The listing builds one solid part. Answer for the finished solid, in the listing's coordinates (mm). A direction names the side the tool comes from. Give positions to 0.01 mm unless a question says otherwise; leave off trailing zeros. Write each loop counter-clockwise with the first axis right and the second up, starting at its lowest first coordinate (ties: lowest second). Pieces come first, ordered by that corner, then holes. Notation, with made-up numbers: M 82.5,36.5 L 114.5,36.5 A14 cw 114.5,51.5 Z; hole C 27,81 d2. An arc over 180 degrees is marked long. Answer as a JSON object with one key per item and string values.
```python
from build123d import *

# Parameters (mm, degrees)
F1_DEPTH = 11
F2_R     = 28.523991
F3_R     = 5
F5_R     = 0.75
F6_DEPTH = 11.001
F7_R     = 4
F8_DEPTH = 11.001


with BuildPart() as f1:
    # F0 (on Top) → F1 (new body)
    with BuildSketch(Plane.XY):
        with BuildLine():
            ThreePointArc((-59.119348, -199.42142), (-183.034682, -98.804378), (-199.158229, 60))
            Line((-199.158229, 60), (-222.036033, 60))
            ThreePointArc((-222.036033, 60), (0, -230), (222.036033, 60))
            Line((222.036033, 60), (199.158229, 60))
            ThreePointArc((199.158229, 60), (183.034682, -98.804378), (59.119348, -199.42142))
            Line((59.119348, -199.42142), (25, -188))
            Line((25, -188), (0, -188))
            Line((0, -188), (-25, -188))
            Line((-25, -188), (-59.119348, -199.42142))
        make_face()
    extrude(amount=F1_DEPTH)

    # F2
    f2_edges = [f1.edges().sort_by_distance(p)[0] for p in [
        (25, -188, 5.5),
        (-25, -188, 5.5),
    ]]
    fillet(f2_edges, radius=F2_R)

    # F3
    f3_edges = [f1.edges().sort_by_distance(p)[0] for p in [
        (59.119348, -199.42142, 5.5),
        (-59.119348, -199.42142, 5.5),
    ]]
    fillet(f3_edges, radius=F3_R)

    # F5 (on face) → F6 (cut, through all)
    with BuildSketch(Plane.XY.offset(11)):
        with Locations((0, -219)):
            Circle(F5_R)
        with Locations((48.732085, -213.509213)):
            Circle(F5_R)
        with Locations((95.020539, -197.312182)):
            Circle(F5_R)
        with Locations((136.544267, -171.221095)):
            Circle(F5_R)
        with Locations((171.221095, -136.544267)):
            Circle(F5_R)
        with Locations((197.312182, -95.020539)):
            Circle(F5_R)
        with Locations((213.509213, -48.732085)):
            Circle(F5_R)
        with Locations((219, 0)):
            Circle(F5_R)
        with Locations((213.509213, 48.732085)):
            Circle(F5_R)
        with Locations((197.312182, 95.020539)):
            Circle(F5_R)
        with Locations((171.221095, 136.544267)):
            Circle(F5_R)
        with Locations((136.544267, 171.221095)):
            Circle(F5_R)
        with Locations((95.020539, 197.312182)):
            Circle(F5_R)
        with Locations((48.732085, 213.509213)):
            Circle(F5_R)
        with Locations((0, 219)):
            Circle(F5_R)
        with Locations((-48.732085, 213.509213)):
            Circle(F5_R)
        with Locations((-95.020539, 197.312182)):
            Circle(F5_R)
        with Locations((-136.544267, 171.221095)):
            Circle(F5_R)
        with Locations((-171.221095, 136.544267)):
            Circle(F5_R)
        with Locations((-197.312182, 95.020539)):
            Circle(F5_R)
        with Locations((-213.509213, 48.732085)):
            Circle(F5_R)
        with Locations((-219, 0)):
            Circle(F5_R)
        with Locations((-213.509213, -48.732085)):
            Circle(F5_R)
        with Locations((-197.312182, -95.020539)):
            Circle(F5_R)
        with Locations((-171.221095, -136.544267)):
            Circle(F5_R)
        with Locations((-136.544267, -171.221095)):
            Circle(F5_R)
        with Locations((-95.020539, -197.312182)):
            Circle(F5_R)
        with Locations((-48.732085, -213.509213)):
            Circle(F5_R)
        with Locations((-5, -197)):
            Circle(F5_R)
        with Locations((5, -197)):
            Circle(F5_R)
        with Locations((0, -208)):
            Circle(F5_R)
        with Locations((-5, -217)):
            Circle(F5_R)
        with Locations((-25, -207)):
            Circle(F5_R)
        with Locations((5, -217)):
            Circle(F5_R)
        with Locations((25, -207)):
            Circle(F5_R)
    extrude(amount=-F6_DEPTH, mode=Mode.SUBTRACT)

    # F7 (on face) → F8 (cut, through all)
    with BuildSketch(Plane.XY.offset(11)):
        with Locations((-171.221095, -136.544267)):
            Circle(F7_R)
        with Locations((171.221095, -136.544267)):
            Circle(F7_R)
    extrude(amount=-F8_DEPTH, mode=Mode.SUBTRACT)


solid = f1.part
```
1. The mould has two halves that part along X. Classify faces 4 (the cylindrical face through (-182.33, -100.1, 5.42)), 5 (the flat face through (-1, -192, 0)), 6 (the flat face through (-43.31, -194.13, 5.42)), 7 (the cylindrical face through (-5.907, -229.924, 5.423)): released by +X, released by -X, zero draft, split by the parting line, or undercut.
Verdict:
{"face 4": "undercut", "face 5": "zero draft", "face 6": "undercut", "face 7": "split by the parting line"}
2. A cutting plane is placed at B-B, the plane y = 41. Give the vertices of the cut face in (x, z).
Verdict:
{"outline": "M -226.32,0 L -203.92,0 L -203.92,11 L -226.32,11 Z; M 203.92,0 L 226.32,0 L 226.32,11 L 203.92,11 Z"}
3. A cutting plane is placed at A-A, the plane y = -77. Give the vertices of the cut face in (x, z).
Verdict:
{"outline": "M -216.73,0 L -193.22,0 L -193.22,11 L -216.73,11 Z; M 193.22,0 L 216.73,0 L 216.73,11 L 193.22,11 Z"}
4. A cutting plane is placed at C-C, the plane x = 148. Give the vertices of the cut face in (y, z).
Verdict:
{"outline": "M -176.06,0 L -146.15,0 L -146.15,11 L -176.06,11 Z"}
5. A cutting plane is placed at D-D, the plane z = 3. Count the separate pieces of the cut face and the enclosed holes in it, plus the area to 3 significant figures.
Verdict:
{"separate pieces": "1", "enclosed holes": "24", "area": "19,300 mm2"}
6. Consider line 1 along Y through (x, z) = (5, 9.25); line 2 along X through (y, z) = (-172.5, 4); line 3 along X through (y, z) = (-151, 7). Determine where each line is inside the solid, lowest interval first.
Verdict:
{"line 1": "y = -229.95 to -217.75, -216.25 to -197.75, -196.25 to -188", "line 2": "x = -152.13 to -116.22, 116.22 to 152.13", "line 3": "x = -173.49 to -143.05, 143.05 to 173.49"}
7. Flat-ended cylindrical pins translate along their axes: pin 1 (5 mm diameter, centred on x = 163, z = 1.5, fed in from -Y); pin 2 (6 mm diameter, centred on x = -117, z = 2, fed in from -Y); pin 3 (5 mm diameter, centred on x = -44, z = 7, fed in from -Y) (3 decimals). Find the tip coordinate at first contact, or state that the pin passes through.
Verdict:
{"pin 1": "stops at y = -164.74", "pin 2": "stops at y = -199.76", "pin 3": "stops at y = -226.225"}
8. For faces 1 (the cylindrical face through (184.48, -96.08, 5.42)), 2 (the flat face through (-210, 60, 5)), 3 (the cylindrical face through (25, -188.38, 5.58)), determine the directions among +Z, -Z, +X, -X, +Y, -Y from which every point of the face is accessible in a straight line to the end or side of a thin tool.
Verdict:
{"face 1": "+Z, -Z", "face 2": "+Z, -Z, +X, -X, +Y", "face 3": "+Z, -Z, +Y"}
